from build123d import *

# Parameters (mm, degrees)
F2_DEPTH = 25.4


with BuildPart() as f2:
    # F1 (on face) → F2 (new body)
    with BuildSketch(Plane.XZ):
        Polygon((-15.739672, 6.558197), (-15.739672, 40.369343), (-27.107213, 40.369343), (-27.107213, 6.558197), (-21.277705, -5.392295), align=None)
    extrude(amount=F2_DEPTH)


solid = f2.part
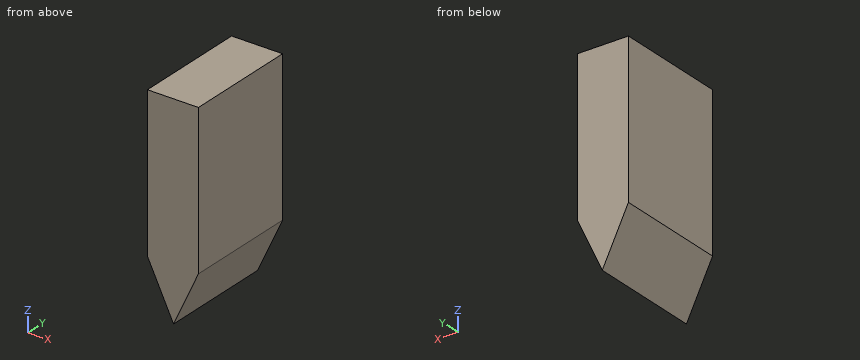
The model under review builds one solid part; all positions refer to its coordinate system, in mm. Round coordinates to 2 decimals unless told otherwise and drop trailing zeros. Order: outer loops, then holes, each group sorted by start corner. A loop starts at its lowest first (then second) coordinate and runs counter-clockwise, first axis right, second up. Notation, with made-up numbers: (45.5, 7.5) - (80.5, 7.5) arc R25 cw to (80.5, 22.5) - close; hole circle Ø4 at (44, -8). An arc over 180 degrees is marked (long way). Use one line per item in the form item = value.
Q1. Add section B-B on x = -17.5. Give the boundary of the cut face in (y, z).
Response values:
outline = (-25.4, 2.76) - (0, 2.76) - (0, 40.37) - (-25.4, 40.37) - close
Q2. Add section A-A on y = -21.25. Give the boundary of the cut face in (x, z).
Response values:
outline = (-27.11, 6.56) - (-21.28, -5.39) - (-15.74, 6.56) - (-15.74, 40.37) - (-27.11, 40.37) - close
Q3. To check wall thickness, follow line 1 (Z direction, x = -26.5, y = -16.5); line 2 (Z direction, x = -19.75, y = -9.5); line 3 (X direction, y = -5.5, z = 6). State the ranges of each line that lie inside material, in increasing order.
Response values:
line_1 = 5.31 to 40.37
line_2 = -2.1 to 40.37
line_3 = -26.83 to -16
Q4. Add section C-C on z = 0. Give the boundary of the cut face in (x, y), then the cut area to 3 significant figures.
Response values:
outline = (-23.91, -25.4) - (-18.78, -25.4) - (-18.78, 0) - (-23.91, 0) - close
area = 130 mm^2
Q5. Clearance check with flat-ended pins moving along their axes: P1, Ø3, axis at x = -20, y = -18, coming from the -Z side; P2, Ø1, axis at x = -20.5, y = -9, coming from the -Z side; P3, Ø5, axis at y = -12, z = 1.5, coming from the -X side. State where each tip first meets the part, or that it passes through.
Response values:
P1 = -5.39
P2 = -4.79
P3 = -25.86
